Here's how the part is built. I have some questions about the finished solid (model axes, mm). A direction names the side the tool comes from. Round coordinates to 2 decimals unless told otherwise and drop trailing zeros. Loops run counter-clockwise (first coordinate to the right, second up) from the corner with the lowest first, then second, coordinate; pieces in that order, holes last. Notation, with made-up numbers: M 13.25,-7 L 58.25,-7 A21 ccw 58.25,2 Z; hole C -16,-4 d7. An arc over 180 degrees is marked long. Answer as CSV lines item,"result".
```python
from build123d import *

# Parameters (mm, degrees)
BOSS_EXTRU_1_DEPTH      = 36
ESQUISSE6_W             = 100
ESQUISSE6_H             = 28
ENL_V_MAT_EXTRU_1_DEPTH = 14
ENL_V_MAT_EXTRU_2_REACH = 152.814
ESQUISSE7_R             = 1.6
ENL_V_MAT_EXTRU_3_REACH = 153.697
ESQUISSE8_R             = 3.1
ENL_V_MAT_EXTRU_4_DEPTH = 5.5


with BuildPart() as part:
    # Esquisse5 → Boss.-Extru.1 (new body)
    with BuildSketch(Plane.XY):
        Polygon((0, 0), (0, 46), (20, 46), (20, 17), (120, 17), (120, 46), (140, 46), (140, 0), align=None)
    extrude(amount=BOSS_EXTRU_1_DEPTH)

    # Esquisse6 → Enlèv. mat.-Extru.1 (cut)
    with BuildSketch(Plane(origin=(0, 17, 0), x_dir=(1, 0, 0), z_dir=(0, 1, 0))):
        with Locations((70, -18)):
            Rectangle(ESQUISSE6_W, ESQUISSE6_H)
    extrude(amount=-ENL_V_MAT_EXTRU_1_DEPTH, mode=Mode.SUBTRACT)

    # Esquisse7 → Enlèv. mat.-Extru.2 (cut, up to next)
    with BuildSketch(Plane(origin=(0, 3, 0), x_dir=(1, 0, 0), z_dir=(0, 1, 0)), mode=Mode.PRIVATE) as enl_v_mat_extru_2_sk1:
        with Locations(Location((36.5, -11, 0), (0, 0, 270))):
            Circle(ESQUISSE7_R)
    enl_v_mat_extru_2_tool1 = extrude(enl_v_mat_extru_2_sk1.sketch, amount=-ENL_V_MAT_EXTRU_2_REACH, mode=Mode.PRIVATE) & part.part
    # Esquisse7 → Enlèv. mat.-Extru.2 (cut, up to next)
    with BuildSketch(Plane(origin=(0, 3, 0), x_dir=(1, 0, 0), z_dir=(0, 1, 0)), mode=Mode.PRIVATE) as enl_v_mat_extru_2_sk2:
        with Locations(Location((97, -11, 0), (0, 0, 270))):
            Circle(ESQUISSE7_R)
    enl_v_mat_extru_2_tool2 = extrude(enl_v_mat_extru_2_sk2.sketch, amount=-ENL_V_MAT_EXTRU_2_REACH, mode=Mode.PRIVATE) & part.part
    # Esquisse7 → Enlèv. mat.-Extru.2 (cut, up to next)
    with BuildSketch(Plane(origin=(0, 3, 0), x_dir=(1, 0, 0), z_dir=(0, 1, 0)), mode=Mode.PRIVATE) as enl_v_mat_extru_2_sk3:
        with Locations(Location((97, -25, 0), (0, 0, 180))):
            Circle(ESQUISSE7_R)
    enl_v_mat_extru_2_tool3 = extrude(enl_v_mat_extru_2_sk3.sketch, amount=-ENL_V_MAT_EXTRU_2_REACH, mode=Mode.PRIVATE) & part.part
    # Esquisse7 → Enlèv. mat.-Extru.2 (cut, up to next)
    with BuildSketch(Plane(origin=(0, 3, 0), x_dir=(1, 0, 0), z_dir=(0, 1, 0)), mode=Mode.PRIVATE) as enl_v_mat_extru_2_sk4:
        with Locations(Location((36.5, -25, 0), (0, 0, 180))):
            Circle(ESQUISSE7_R)
    enl_v_mat_extru_2_tool4 = extrude(enl_v_mat_extru_2_sk4.sketch, amount=-ENL_V_MAT_EXTRU_2_REACH, mode=Mode.PRIVATE) & part.part
    add(enl_v_mat_extru_2_tool1.solids().sort_by_distance((36.5, 3, 11))[0], mode=Mode.SUBTRACT)
    add(enl_v_mat_extru_2_tool2.solids().sort_by_distance((97, 3, 11))[0], mode=Mode.SUBTRACT)
    add(enl_v_mat_extru_2_tool3.solids().sort_by_distance((97, 3, 25))[0], mode=Mode.SUBTRACT)
    add(enl_v_mat_extru_2_tool4.solids().sort_by_distance((36.5, 3, 25))[0], mode=Mode.SUBTRACT)

    # Esquisse8 → Enlèv. mat.-Extru.3 (cut, up to next)
    with BuildSketch(Plane(origin=(0, 46, 0), x_dir=(1, 0, 0), z_dir=(0, 1, 0)), mode=Mode.PRIVATE) as enl_v_mat_extru_3_sk1:
        with Locations(Location((10, -8, 0), (0, 0, 270))):
            Circle(ESQUISSE8_R)
    enl_v_mat_extru_3_tool1 = extrude(enl_v_mat_extru_3_sk1.sketch, amount=-ENL_V_MAT_EXTRU_3_REACH, mode=Mode.PRIVATE) & part.part
    # Esquisse8 → Enlèv. mat.-Extru.3 (cut, up to next)
    with BuildSketch(Plane(origin=(0, 46, 0), x_dir=(1, 0, 0), z_dir=(0, 1, 0)), mode=Mode.PRIVATE) as enl_v_mat_extru_3_sk2:
        with Locations(Location((10, -28, 0), (0, 0, 270))):
            Circle(ESQUISSE8_R)
    enl_v_mat_extru_3_tool2 = extrude(enl_v_mat_extru_3_sk2.sketch, amount=-ENL_V_MAT_EXTRU_3_REACH, mode=Mode.PRIVATE) & part.part
    # Esquisse8 → Enlèv. mat.-Extru.3 (cut, up to next)
    with BuildSketch(Plane(origin=(0, 46, 0), x_dir=(1, 0, 0), z_dir=(0, 1, 0)), mode=Mode.PRIVATE) as enl_v_mat_extru_3_sk3:
        with Locations(Location((130, -28, 0), (0, 0, 180))):
            Circle(ESQUISSE8_R)
    enl_v_mat_extru_3_tool3 = extrude(enl_v_mat_extru_3_sk3.sketch, amount=-ENL_V_MAT_EXTRU_3_REACH, mode=Mode.PRIVATE) & part.part
    # Esquisse8 → Enlèv. mat.-Extru.3 (cut, up to next)
    with BuildSketch(Plane(origin=(0, 46, 0), x_dir=(1, 0, 0), z_dir=(0, 1, 0)), mode=Mode.PRIVATE) as enl_v_mat_extru_3_sk4:
        with Locations(Location((130, -8, 0), (0, 0, 180))):
            Circle(ESQUISSE8_R)
    enl_v_mat_extru_3_tool4 = extrude(enl_v_mat_extru_3_sk4.sketch, amount=-ENL_V_MAT_EXTRU_3_REACH, mode=Mode.PRIVATE) & part.part
    add(enl_v_mat_extru_3_tool1.solids().sort_by_distance((10, 46, 8))[0], mode=Mode.SUBTRACT)
    add(enl_v_mat_extru_3_tool2.solids().sort_by_distance((10, 46, 28))[0], mode=Mode.SUBTRACT)
    add(enl_v_mat_extru_3_tool3.solids().sort_by_distance((130, 46, 28))[0], mode=Mode.SUBTRACT)
    add(enl_v_mat_extru_3_tool4.solids().sort_by_distance((130, 46, 8))[0], mode=Mode.SUBTRACT)

    # Esquisse9 → Enlèv. mat.-Extru.4 (cut)
    with BuildSketch(Plane.XZ):
        Polygon((124.9, 5.055513627), (130, 2.111027254), (135.1, 5.055513627), (135.1, 10.944486373), (130, 13.888972746), (124.9, 10.944486373), align=None)
        Polygon((124.9, 25.055513627), (124.9, 30.944486373), (130, 33.888972746), (135.1, 30.944486373), (135.1, 25.055513627), (130, 22.111027254), align=None)
        Polygon((15.1, 30.944486373), (10, 33.888972746), (4.9, 30.944486373), (4.9, 25.055513627), (10, 22.111027254), (15.1, 25.055513627), align=None)
        Polygon((15.1, 10.944486373), (15.1, 5.055513627), (10, 2.111027254), (4.9, 5.055513627), (4.9, 10.944486373), (10, 13.888972746), align=None)
    extrude(amount=-ENL_V_MAT_EXTRU_4_DEPTH, mode=Mode.SUBTRACT)


solid = part.part
```
1. I want a section at D-D, the plane y = 8. Please give me the cut outline in (x, z), and give its area (3 significant figures).
Evaluation:
outline,"M 0,0 L 140,0 L 140,36 L 0,36 Z; hole C 10,8 d6.2; hole C 10,28 d6.2; hole M 20,4 L 120,4 L 120,32 L 20,32 Z; hole C 130,8 d6.2; hole C 130,28 d6.2"
area,"2,120 mm²"
2. We'd pull the mould along Z, two halves only. Please class faces 4 (the flat face through (69, 17, 34)), 5 (the flat face through (12.51, 2.71, 12.44)): pulls with the +Z half, pulls with the -Z half, needs draft (parallel to the pull), parting line crosses it, or undercut.
Evaluation:
face 4,"needs draft"
face 5,"undercut"
3. I want a section at C-C, the plane z = 8. Please give me the cut outline in (x, y), and give its area (3 significant figures).
Evaluation:
outline,"M 0,0 L 4.9,0 L 4.9,5.5 L 6.9,5.5 L 6.9,46 L 0,46 Z; M 13.1,5.5 L 15.1,5.5 L 15.1,0 L 124.9,0 L 124.9,5.5 L 126.9,5.5 L 126.9,46 L 120,46 L 120,3 L 20,3 L 20,46 L 13.1,46 Z; M 133.1,5.5 L 135.1,5.5 L 135.1,0 L 140,0 L 140,46 L 133.1,46 Z"
area,"1,530 mm²"
4. I want a section at B-B, the plane y = 42.5. Please give me the cut outline in (x, z).
Evaluation:
outline,"M 0,0 L 20,0 L 20,36 L 0,36 Z; M 120,0 L 140,0 L 140,36 L 120,36 Z; hole C 10,8 d6.2; hole C 10,28 d6.2; hole C 130,8 d6.2; hole C 130,28 d6.2"
5. Which directions (+Z, -Z, +X, -X, +Y, -Y) give clear straight access to the entire face, cutting with the end or side of a thin tool? Please do faces 1 (the flat face through (69, 17, 2)), 2 (the flat face through (120, 24, 18)), 3 (the flat face through (4.9, 3, 8)).
Evaluation:
face 1,"+Z, -Z, +Y"
face 2,"+Y"
face 3,"-Y"
6. For P1, Ø5, axis at x = 130, z = 8, coming from the -Y side; P2, Ø8, axis at x = 130, z = 28, coming from the -Y side; P3, Ø4.5, axis at x = 64, z = 1.5, coming from the +Y side; P4, Ø1.5, axis at x = 110, z = 29, coming from the +Y side, each with a flat end and sliding along its axis, tell me the tip position at first contact or that it passes through.
Evaluation:
P1,"passes through"
P2,"stops at y = 5.5"
P3,"stops at y = 17"
P4,"stops at y = 3"
7. I want a section at A-A, the plane x = 97. Please give me the cut outline in (y, z), and give its area (3 significant figures).
Evaluation:
outline,"M 0,0 L 17,0 L 17,4 L 3,4 L 3,9.4 L 0,9.4 Z; M 0,12.6 L 3,12.6 L 3,23.4 L 0,23.4 Z; M 0,26.6 L 3,26.6 L 3,32 L 17,32 L 17,36 L 0,36 Z"
area,"201 mm²"
8. If I drill on line 1 (Z direction, x = 97, y = 0.8); line 2 (Z direction, x = 130, y = 16); line 3 (X direction, y = 9, z = 23), over which ranges is the centre line in solid material (lowest first)? Write a range as [from, to].
Evaluation:
line 1,"z = [0, 9.4], [12.6, 23.4], [26.6, 36]"
line 2,"z = [0, 4.9], [11.1, 24.9], [31.1, 36]"
line 3,"x = [0, 20], [120, 140]"
